from build123d import *

# Parameters (mm, degrees)
SKETCH1_R                       = 1.016
BOSS_EXTRUDE1_DEPTH             = 2
SKETCH2_R                       = 4.7
BOSS_EXTRUDE2_DEPTH             = 3
BOSS_EXTRUDE5_DEPTH             = 8
BOSS_EXTRUDE6_REACH             = 53.49
BOSS_EXTRUDE6_DIRECTION_2_REACH = 53.49
SKETCH4_W                       = 22.5
SKETCH4_H                       = 14.127681706
CUT_EXTRUDE1_DEPTH              = 7
FILLET1_R                       = 0.5
SKETCH5_R                       = 2.5
BOSS_EXTRUDE7_DEPTH             = 1
SKETCH6_W                       = 5.313656685
SKETCH6_H                       = 4.599259183
SKETCH6_W_2                     = 16.163165117
SKETCH6_H_2                     = 5.344557169
CUT_EXTRUDE2_DEPTH              = 5


with BuildPart() as part:
    # Sketch1 → Boss-Extrude1 (new body)
    # profile 1 of 4: a face of its own
    with BuildSketch(Plane.XY):
        with BuildLine():
            Line((-16.05, 5.25), (-16.05, -5.25))
            ThreePointArc((-16.05, -5.25), (-15.801040764, -5.851040764), (-15.2, -6.1))
            Line((-15.2, -6.1), (-11.25, -6.1))
            Line((-11.25, -6.1), (-11.25, 6.1))
            Line((-11.25, 6.1), (-15.2, 6.1))
            ThreePointArc((-15.2, 6.1), (-15.801040764, 5.851040764), (-16.05, 5.25))
        make_face()
        with Locations((-13.9, 0)):
            Circle(SKETCH1_R, mode=Mode.SUBTRACT)
    # profile 2 of 4: a face of its own
    with BuildSketch(Plane.XY):
        with BuildLine():
            Line((16.05, 5.25), (16.05, -5.25))
            ThreePointArc((16.05, -5.25), (15.801040764, -5.851040764), (15.2, -6.1))
            Line((15.2, -6.1), (11.25, -6.1))
            Line((11.25, -6.1), (11.25, 6.094097151))
            Line((11.25, 6.094097151), (15.2, 6.1))
            ThreePointArc((15.2, 6.1), (15.801040764, 5.851040764), (16.05, 5.25))
        make_face()
        with Locations((13.9, 0)):
            Circle(SKETCH1_R, mode=Mode.SUBTRACT)
    # profile 3 of 4: a face of its own
    with BuildSketch(Plane.XY):
        with BuildLine():
            ThreePointArc((15.2, -6.1), (15.801040764, -5.851040764), (16.05, -5.25))
            Line((16.05, -5.25), (16.05, -6.1))
            Line((16.05, -6.1), (15.2, -6.1))
        make_face()
    # profile 4 of 4: a face of its own
    with BuildSketch(Plane.XY):
        with BuildLine():
            ThreePointArc((-16.05, -5.25), (-15.801040764, -5.851040764), (-15.2, -6.1))
            Line((-15.2, -6.1), (-16.05, -6.1))
            Line((-16.05, -6.1), (-16.05, -5.25))
        make_face()
    extrude(amount=BOSS_EXTRUDE1_DEPTH)

    # Sketch2 → Boss-Extrude2 (add)
    with BuildSketch(Plane.XZ.offset(6.1)):
        Polygon((16.05, 2), (11.25, 2), (11.25, 38.372960525), (-1.65, 41.317302208), (-1.65, 22.612965014), (-1.65, 2), (-16.05, 2), (-16.05, 0), (-1.65, 0), (-1.65, -32.240273927), (11.25, -31.043279545), (11.25, 0), (16.05, 0), align=None)
        with Locations((4.75, -19)):
            Circle(SKETCH2_R, mode=Mode.SUBTRACT)
    extrude(amount=BOSS_EXTRUDE2_DEPTH)

    # Sketch2<3> → Boss-Extrude5 (add)
    with BuildSketch(Plane.XZ.offset(6.1)):
        with BuildLine():
            ThreePointArc((7.17535625, 36.893660937), (9.334777443, 36.079294831), (11.25, 34.791578013))
            Line((11.25, 34.791578013), (11.25, 38.372960525))
            Line((11.25, 38.372960525), (-1.65, 41.317302208))
            Line((-1.65, 41.317302208), (-1.65, 39.1))
            Line((-1.65, 39.1), (7.17535625, 36.893660937))
        make_face()
        with BuildLine():
            ThreePointArc((0.350023778, -29.2), (-0.651218811, -29.175170712), (-1.65, -29.100743889))
            Line((-1.65, -29.100743889), (-1.65, -32.240273927))
            Line((-1.65, -32.240273927), (11.25, -31.043279545))
            Line((11.25, -31.043279545), (11.25, -26.86066155))
            ThreePointArc((11.25, -26.86066155), (8.204073841, -28.597362862), (4.75, -29.2))
            Line((4.75, -29.2), (0.350023778, -29.2))
        make_face()
    extrude(amount=BOSS_EXTRUDE5_DEPTH)

    # Boss-Extrude6: up to this face of the body (flat: up to its plane)
    boss_extrude6_end = Plane(part.part.faces().sort_by_distance((16.05, -1.925, 1))[0])
    # Sketch3 → Boss-Extrude6 (add, up to the picked face)
    with BuildSketch(Plane(origin=(11.25, 0, 0), x_dir=(0, 0, -1), z_dir=(1, 0, 0)), mode=Mode.PRIVATE) as boss_extrude6_sk1:
        Polygon((-7.665828596, -9.1), (-2, -3.457464127), (-2, -9.1), align=None)
    boss_extrude6_tool1 = split(extrude(boss_extrude6_sk1.sketch, amount=BOSS_EXTRUDE6_REACH, mode=Mode.PRIVATE), bisect_by=boss_extrude6_end, keep=Keep.BOTH, mode=Mode.PRIVATE)
    add(boss_extrude6_tool1.solids().sort_by(Axis((11.25, -7.219155, 3.88861), (1, 0, 0)))[0])

    # Boss-Extrude6 direction 2: up to this face of the body (flat: up to its plane)
    boss_extrude6_direction_2_end = Plane(part.part.faces().sort_by_distance((-16.05, -1.925, 1))[0])
    # Sketch3 → Boss-Extrude6 direction 2 (add, up to the picked face)
    with BuildSketch(Plane(origin=(11.25, 0, 0), x_dir=(0, 0, -1), z_dir=(1, 0, 0)), mode=Mode.PRIVATE) as boss_extrude6_direction_2_sk1:
        Polygon((-7.665828596, -9.1), (-2, -3.457464127), (-2, -9.1), align=None)
    boss_extrude6_direction_2_tool1 = split(extrude(boss_extrude6_direction_2_sk1.sketch, amount=-BOSS_EXTRUDE6_DIRECTION_2_REACH, mode=Mode.PRIVATE), bisect_by=boss_extrude6_direction_2_end, keep=Keep.BOTH, mode=Mode.PRIVATE)
    add(boss_extrude6_direction_2_tool1.solids().sort_by(Axis((11.25, -7.219155, 3.88861), (-1, 0, 0)))[0])

    # Sketch4 → Cut-Extrude1 (cut)
    with BuildSketch(Plane(origin=(0, -6.1, 0), x_dir=(1, 0, 0), z_dir=(0, 1, 0))):
        with Locations((0, -7.063840853)):
            Rectangle(SKETCH4_W, SKETCH4_H)
    extrude(amount=CUT_EXTRUDE1_DEPTH, mode=Mode.SUBTRACT)

    # Fillet1
    fillet1_edges = [part.edges().sort_by_distance(p)[0] for p in [
        (13.65, -9.1, 7.665828596),
        (-8.85, -9.1, 7.665828596),
    ]]
    fillet(fillet1_edges, radius=FILLET1_R)

    # Sketch5 → Boss-Extrude7 (add)
    with BuildSketch(Plane.XZ.offset(9.1)):
        with BuildLine():
            Line((-1.65, 39.1), (-1.65, 6.455196792))
            Line((-1.65, 6.455196792), (-16.05, 6.455196792))
            Line((-16.05, 6.455196792), (-16.05, 0))
            Line((-16.05, 0), (-1.65, 0))
            Line((-1.65, 0), (-1.65, -29.100743889))
            ThreePointArc((-1.65, -29.100743889), (-0.651218811, -29.175170712), (0.350023778, -29.2))
            Line((0.350023778, -29.2), (4.75, -29.2))
            ThreePointArc((4.75, -29.2), (8.204073841, -28.597362862), (11.25, -26.86066155))
            Line((11.25, -26.86066155), (11.25, 0))
            Line((11.25, 0), (16.05, 0))
            Line((16.05, 0), (16.05, 6.455196792))
            Line((16.05, 6.455196792), (11.25, 6.455196792))
            Line((11.25, 6.455196792), (11.25, 34.791578013))
            ThreePointArc((11.25, 34.791578013), (9.334777443, 36.079294831), (7.17535625, 36.893660937))
            Line((7.17535625, 36.893660937), (-1.65, 39.1))
        make_face()
        with Locations((4.75, -19)):
            Circle(SKETCH5_R, mode=Mode.SUBTRACT)
    extrude(amount=BOSS_EXTRUDE7_DEPTH)

    # Sketch6 → Cut-Extrude2 (cut)
    with BuildSketch(Plane.XY.offset(6.455196792)):
        with Locations((13.906828343, -7.800370409)):
            Rectangle(SKETCH6_W, SKETCH6_H)
        with Locations((-9.731582558, -7.427721416)):
            Rectangle(SKETCH6_W_2, SKETCH6_H_2)
    extrude(amount=CUT_EXTRUDE2_DEPTH, mode=Mode.SUBTRACT)


solid = part.part
Geometry: final body of the model. Coordinates: model frame, mm. A direction names the side the tool comes from. Give positions to 0.01 mm unless a question says otherwise; leave off trailing zeros. Order: outer loops, then holes, each group sorted by start corner. A loop starts at its lowest first (then second) coordinate and runs counter-clockwise, first axis right, second up. Notation, with made-up numbers: (74.25, 56) -> (97.25, 56) arc R20 cw to (97.25, 75) -> close; hole circle Ø1 at (-14, -12.5). An arc over 180 degrees is marked (long way). Answer as a JSON object with one key per item and string values.
Q1. First-contact query: pin 1 (1 mm diameter, centred on y = -5, z = -15, fed in from +X); pin 2 (4 mm diameter, centred on y = -9.5, z = -16, fed in from +X); pin 3 (5 mm diameter, centred on x = 6.5, y = -7, fed in from +Z); pin 4 (9 mm diameter, centred on y = -8.5, z = 27.5, fed in from -X). Flat tips, straight axial feed; report the tip coordinate or a pass-through.
Entries:
{"pin 1": "passes through", "pin 2": "stops at x = 11.25", "pin 3": "stops at z = 40.03", "pin 4": "stops at x = -1.65"}
Q2. Access query for faces 5 (the cylindrical face through (8.25, -12.07, -28.58)), 6 (the flat face through (11.25, 0, 1)), 7 (the flat face through (13.7, 1.4, 2)). Directions: +Z, -Z, +X, -X, +Y, -Y. A direction counts if a zero-diameter tool reaches every point of the face in a straight line with its end or side. Return the directions, or none.
Entries:
{"face 5": "-Y", "face 6": "+Z, -Z, +Y", "face 7": "+Z, +X, -X, +Y"}
Q3. Draft query along Y for faces 1 (the flat face through (-10.551, -6.693, 5.249)), 2 (the flat face through (3, -10.1, 5)), 3 (the cylindrical face through (-0.637, -12.072, -29.176)), 4 (the cylindrical face through (12.885, 0.045, 0.986)). Return one class per face: released by +Y, released by -Y, zero draft, split by the parting line, or undercut.
Entries:
{"face 1": "released by +Y", "face 2": "released by -Y", "face 3": "zero draft", "face 4": "undercut"}
Q4. Section C-C (z = -19). Output: boundary loops of the cut face in (x, y), plus the area to 3 significant figures.
Entries:
{"outline": "(-1.65, -10.1) -> (2.25, -10.1) -> (2.25, -9.1) -> (0.05, -9.1) -> (0.05, -6.1) -> (-1.65, -6.1) -> close; (7.25, -10.1) -> (11.25, -10.1) -> (11.25, -6.1) -> (9.45, -6.1) -> (9.45, -9.1) -> (7.25, -9.1) -> close", "area": "18.4 mm^2"}
Q5. Section D-D (y = 0). Output: boundary loops of the cut face in (x, z).
Entries:
{"outline": "(-16.05, 0) -> (-14.92, 0) -> (-14.92, 2) -> (-16.05, 2) -> close; (-12.88, 0) -> (-11.25, 0) -> (-11.25, 2) -> (-12.88, 2) -> close; (11.25, 0) -> (12.88, 0) -> (12.88, 2) -> (11.25, 2) -> close; (14.92, 0) -> (16.05, 0) -> (16.05, 2) -> (14.92, 2) -> close"}
Q6. Section A-A (x = -13.9). Output: boundary loops of the cut face in (y, z).
Entries:
{"outline": "(-10.1, 0) -> (-1.02, 0) -> (-1.02, 2) -> (-3.46, 2) -> (-7.89, 6.46) -> (-10.1, 6.46) -> close; (1.02, 0) -> (6.1, 0) -> (6.1, 2) -> (1.02, 2) -> close"}
Q7. Material intervals for probe 1 along Z at (x, y) = (6, -11); probe 2 along Y at (x, z) = (4.5, -3.5); probe 3 along Y at (x, z) = (10.5, -28), sorted ascending.
Entries:
{"probe 1": "z = -31.53 to -29.12, 37.19 to 39.57", "probe 2": "y = -10.1 to -6.1", "probe 3": "y = -14.1 to -6.1"}
Q8. Section B-B (y = -11.25). Output: boundary loops of the cut face in (x, z).
Entries:
{"outline": "(-1.65, -32.24) -> (11.25, -31.04) -> (11.25, -26.86) arc R10.2 cw to (4.75, -29.2) -> (0.35, -29.2) arc R20.2 cw to (-1.65, -29.1) -> close; (-1.65, 39.1) -> (7.18, 36.89) arc R10 cw to (11.25, 34.79) -> (11.25, 38.37) -> (-1.65, 41.32) -> close"}
